Read the model definition and answer for the solid it produces. Units are mm, in the model's axes. Coordinates: 2 decimals unless noted, no trailing zeros. Order: outer loops, then holes, each group sorted by start corner. A loop starts at its lowest first (then second) coordinate and runs counter-clockwise, first axis right, second up. Notation, with made-up numbers: M -33.5,60 L -20.5,60 A29 ccw -20.5,88 Z; hole C 16,0.25 d9. An arc over 180 degrees is marked long. One line per question, with ' | ' between items. Start each with the question number.
1) Find section B-B, the plane z = -30. Write down the section's boundary in (x, y), plus the area to 3 significant figures.
2) Find section A-A, the plane x = 37. Write down the section's boundary in (y, z).
3) Consider probe 1 along Y at (x, z) = (6, 32); probe 2 along Y at (x, z) = (-16, 2); probe 3 along Z at (x, y) = (26, 43). Determine where each line is inside the solid, lowest interval first.
4) Find section C-C, the plane y = 46. Write down the section's boundary in (x, z).
5) Given P1, Ø2, axis at x = -1, y = 29.5, coming from the +Z side; P2, Ø8, axis at x = -17.5, z = 4.5, coming from the +Y side; P3, Ø5, axis at x = -4, z = -17, coming from the +Y side, each flat-ended and moving along its own axis, determine where each tip first touches the part or whether it passes through.
Autodesk Fusion 360 part; units mm, degrees
sketch "Sketch1" plane through (0, 0, 0) normal (1, 0, 0) x (0, 0, -1)
  arc A0 (37.5, 33.0719) -> (-37.5, 33.0719) centre (0, 0) ccw
  line L0 (-37.5, 33.0719) -> (-37.5, 0)
  line L1 (-37.5, 0) -> (37.5, 0)
  line L2 (37.5, 0) -> (37.5, 33.0719)
  dimension "d1" = 50
  dimension "d2" = 75
extrude "Extrude1" add sketch "Sketch1" along normal mid plane 100
chamfer "Chamfer1" distance 5 angle 45 2 edges at (0, 33.0719, 37.5) (0, 33.0719, -37.5)
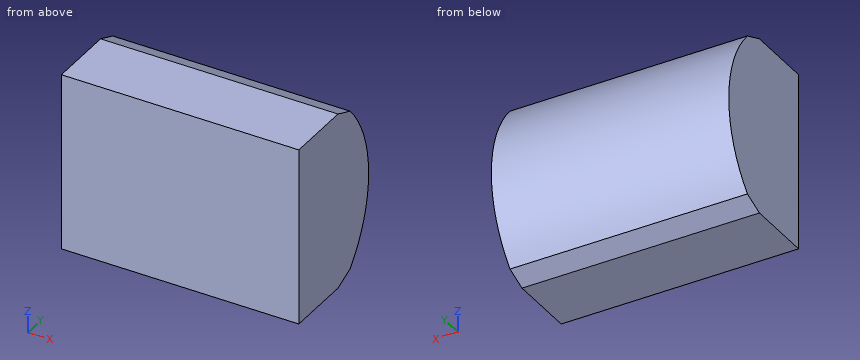
Report:
1) outline: M -50,0 L 50,0 L 50,40 L -50,40 Z | area: 4,000 mm^2
2) outline: M 0,-37.5 L 28.07,-37.5 L 36.65,-34.01 A50 ccw 36.65,34.01 L 28.07,37.5 L 0,37.5 Z
3) probe 1: y = 0 to 38.42 | probe 2: y = 0 to 49.96 | probe 3: z = -25.51 to 25.51
4) outline: M -50,-19.6 L 50,-19.6 L 50,19.6 L -50,19.6 Z
5) P1: stops at z = 37.33 | P2: stops at y = 50 | P3: stops at y = 47.85
